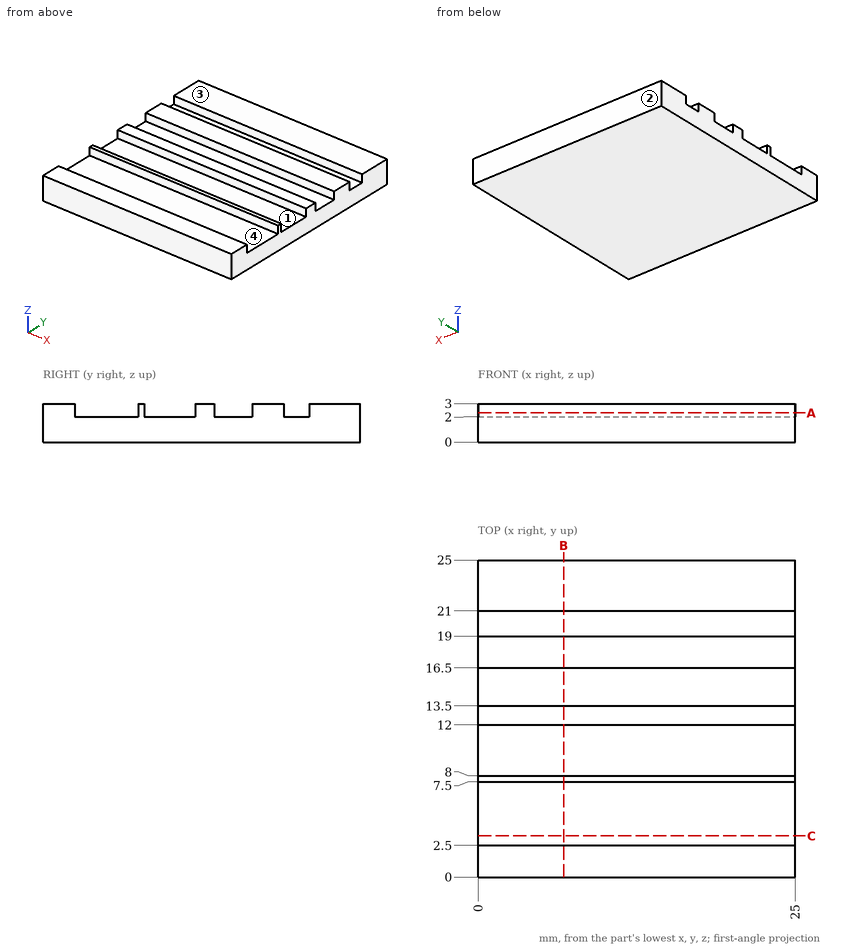
Here's the drawing with two shaded views (mm, measured from the low corner). I have some questions. Round coordinates to 2 decimals unless told otherwise and drop trailing zeros. Write each loop counter-clockwise with the first axis right and the second up, starting at its lowest first coordinate (ties: lowest second). Pieces come first, ordered by that corner, then holes. Notation, with made-up numbers: M -18.75,-38 L 15.25,-38 A25 cw 15.25,-25 Z; hole C -40,-12.75 d1. An arc over 180 degrees is marked long. Use CSV: the item, a comma, the result in double quotes.
(1) We'd pull the mould along Y, two halves only. Please class the marked faces 1, 2, 3 and 4: +Y half, -Y half, draft (parallel to the pull), parting line (faces both ways), or undercut.
Check values:
face 1,"undercut"
face 2,"+Y half"
face 3,"draft"
face 4,"undercut"
(2) Imagine slicing it at B-B (x = 6.75). Write out the boundary of the cut face in (y, z).
Check values:
outline,"M 0,0 L 25,0 L 25,3 L 21,3 L 21,2 L 19,2 L 19,3 L 16.5,3 L 16.5,2 L 13.5,2 L 13.5,3 L 12,3 L 12,2 L 8,2 L 8,3 L 7.5,3 L 7.5,2 L 2.5,2 L 2.5,3 L 0,3 Z"
(3) Imagine slicing it at C-C (y = 3.25). Write out the boundary of the cut face in (x, z).
Check values:
outline,"M 0,0 L 25,0 L 25,2 L 0,2 Z"
(4) Imagine slicing it at A-A (z = 2.3). Write out the boundary of the cut face in (x, y), plus the area to 3 significant figures.
Check values:
outline,"M 0,0 L 25,0 L 25,2.5 L 0,2.5 Z; M 0,7.5 L 25,7.5 L 25,8 L 0,8 Z; M 0,12 L 25,12 L 25,13.5 L 0,13.5 Z; M 0,16.5 L 25,16.5 L 25,19 L 0,19 Z; M 0,21 L 25,21 L 25,25 L 0,25 Z"
area,"275 mm^2"
(5) I'm going to push flat-ended pins straight in: pin 1 (4 mm diameter, centred on x = 2.5, y = 4.5, fed in from -Z); pin 2 (0.9 mm diameter, centred on x = 6.5, y = 15, fed in from +Z). Where does each tip first touch, or does it pass through?
Check values:
pin 1,"z = 0"
pin 2,"z = 2"
(6) I need wall thicknesses on line 1 along Y through (x, z) = (12, 2.25); line 2 along Z through (x, y) = (21.75, 6.5). Which ranges of each line are inside material? Lowest first, please.
Check values:
line 1,"0 to 2.5, 7.5 to 8, 12 to 13.5, 16.5 to 19, 21 to 25"
line 2,"0 to 2"
